Input: dimensioned drawing with shaded views. Units: mm. Origin: part minimum x, y, z. A direction names the side the tool comes from. Coordinates: 2 decimals unless noted, no trailing zeros. Loops run counter-clockwise (first coordinate to the right, second up) from the corner with the lowest first, then second, coordinate; pieces in that order, holes last. Notation, with made-up numbers: (-31, 6.25) - (25, 6.25) arc R8 cw to (25, 20.25) - close; hole circle Ø10 at (-16, 58). An arc over 180 degrees is marked (long way). Put each result on its own line as item: value. Start each with the question number.
1) Material intervals for line 1 along Z through (x, y) = (128.7, 36.85); line 2 along Y through (x, z) = (120, 29); line 3 along X through (y, z) = (19, 17), sorted ascending. Write a range as from..to.
2) Draft query along X for the marked faces 3, 4 and 5. Return one class per face: +X half, -X half, draft (parallel to the pull), parting line (faces both ways), or undercut.
3) Contact query for flat-ended pins moving along their axis: pin 1 Ø12 at (y, z) = (28, 31.5) entering from -X; pin 2 Ø10 at (y, z) = (7, 40.5) entering from -X; pin 3 Ø8 at (x, z) = (163.5, 56) entering from +Y. Output: stop coordinate, or through.
4) Section B-B on y = 9.5. Output: boundary loops of the cut face in (x, z).
5) Section D-D on y = 35.5. Output: boundary loops of the cut face in (x, z), and give its area (3 significant figures).
6) Section C-C on z = 13. Output: boundary loops of the cut face in (x, y).
7) Reachability of the marked faces 1 and 2 from +Z, -Z, +X, -X, +Y, -Y: full face, straight path, thin tool, end or side. Return the list, or none.
8) Section A-A on x = 64.7. Output: boundary loops of the cut face in (y, z).
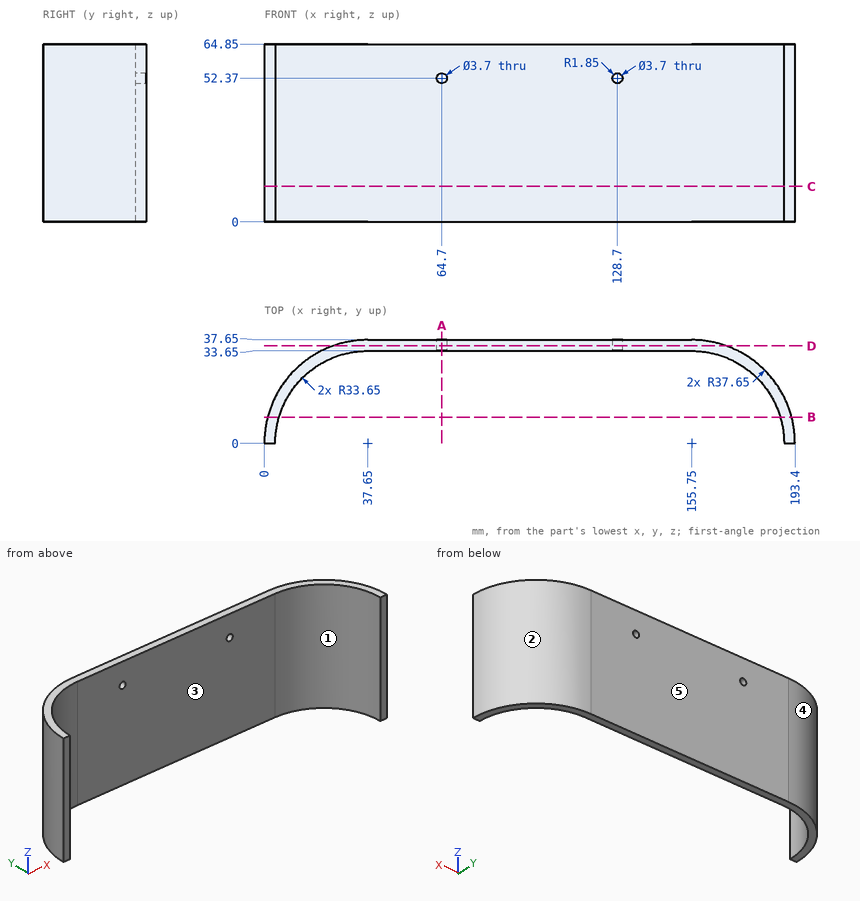
Answer block:
1. line 1: z = 0..50.52, 54.22..64.85
1. line 2: y = 33.65..37.65
1. line 3: x = 5.15..9.88, 183.52..188.25
2. face 3: undercut
2. face 4: -X half
2. face 5: draft
3. pin 1: stops at x = 7.1
3. pin 2: stops at x = 0.05
3. pin 3: stops at y = 37.46
4. outline: (1.22, 0) - (5.37, 0) - (5.37, 64.85) - (1.22, 64.85) - close; (188.03, 0) - (192.18, 0) - (192.18, 64.85) - (188.03, 64.85) - close
5. outline: (25.11, 0) - (168.29, 0) - (168.29, 64.85) - (25.11, 64.85) - close; hole circle Ø3.7 at (64.7, 52.37); hole circle Ø3.7 at (128.7, 52.37)
5. area: 9,260 mm²
6. outline: (0, 0) - (4, 0) arc R33.65 cw to (37.65, 33.65) - (155.75, 33.65) arc R33.65 cw to (189.4, 0) - (193.4, 0) arc R37.65 ccw to (155.75, 37.65) - (37.65, 37.65) arc R37.65 ccw to start
7. face 1: +Z, -Z, -Y
7. face 2: +Z, -Z, +X, +Y
8. outline: (33.65, 0) - (37.65, 0) - (37.65, 50.52) - (33.65, 50.52) - close; (33.65, 54.22) - (37.65, 54.22) - (37.65, 64.85) - (33.65, 64.85) - close
